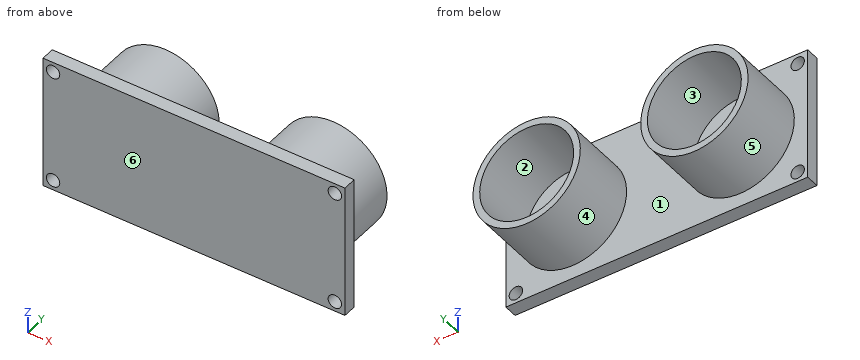
```python
from build123d import *

# Parameters (mm, degrees)
SKETCH1_W           = 45
SKETCH1_H           = 20
SKETCH1_R           = 1
SKETCH1_R_2         = 8
SKETCH1_R_3         = 7
BOSS_EXTRUDE1_DEPTH = 2
SKETCH2_R           = 8
SKETCH2_R_2         = 7
BOSS_EXTRUDE2_DEPTH = 12


with BuildPart() as part:
    # Sketch1 → Boss-Extrude1 (new body)
    with BuildSketch(Plane(origin=(0, 0, 0), x_dir=(1, 0, 0), z_dir=(0, 1, 0))):
        Rectangle(SKETCH1_W, SKETCH1_H)
        with Locations(Location((-21, -8.5, 0), (0, 0, 270))):
            Circle(SKETCH1_R, mode=Mode.SUBTRACT)
        with Locations(Location((-21, 8.5, 0), (0, 0, 270))):
            Circle(SKETCH1_R, mode=Mode.SUBTRACT)
        with Locations((-12.5, 0)):
            Circle(SKETCH1_R_2, mode=Mode.SUBTRACT)
        with Locations(Location((21, -8.5, 0), (0, 0, 270))):
            Circle(SKETCH1_R, mode=Mode.SUBTRACT)
        with Locations(Location((21, 8.5, 0), (0, 0, 270))):
            Circle(SKETCH1_R, mode=Mode.SUBTRACT)
        with Locations((12.5, 0)):
            Circle(SKETCH1_R_2, mode=Mode.SUBTRACT)
        with Locations((-12.5, 0)):
            Circle(SKETCH1_R_2)
        with Locations((-12.5, 0)):
            Circle(SKETCH1_R_3, mode=Mode.SUBTRACT)
        with Locations((-12.5, 0)):
            Circle(SKETCH1_R_3)
        with Locations((12.5, 0)):
            Circle(SKETCH1_R_2)
        with Locations((12.5, 0)):
            Circle(SKETCH1_R_3, mode=Mode.SUBTRACT)
        with Locations((12.5, 0)):
            Circle(SKETCH1_R_3)
    extrude(amount=BOSS_EXTRUDE1_DEPTH)

    # Sketch2 → Boss-Extrude2 (add)
    with BuildSketch(Plane(origin=(0, 0, 0), x_dir=(1, 0, 0), z_dir=(0, 1, 0))):
        with Locations(Location((-12.5, 0, 0), (0, 0, 270))):
            Circle(SKETCH2_R)
        with Locations(Location((-12.5, 0, 0), (0, 0, 270))):
            Circle(SKETCH2_R_2, mode=Mode.SUBTRACT)
        with Locations(Location((12.5, 0, 0), (0, 0, 270))):
            Circle(SKETCH2_R)
        with Locations(Location((12.5, 0, 0), (0, 0, 270))):
            Circle(SKETCH2_R_2, mode=Mode.SUBTRACT)
    extrude(amount=BOSS_EXTRUDE2_DEPTH)


solid = part.part
```
Read the model definition and answer for the solid it produces. Units are mm, in the model's axes. Face numbers are marked on the shaded views. A direction names the side the tool comes from. Coordinates: 2 decimals unless noted, no trailing zeros. Loops run counter-clockwise (first coordinate to the right, second up) from the corner with the lowest first, then second, coordinate; pieces in that order, holes last.
(1) The mould has two halves that part along Z. Classify the marked faces 1, 2, 3 and 4: released by +Z, released by -Z, zero draft, split by the parting line, or undercut.
Solution:
face 1: zero draft
face 2: undercut
face 3: undercut
face 4: split by the parting line
(2) The part is cut by section D-D (z = 0). Determine the outline of the cut face in (x, y).
Solution:
outline: (-22.5, 0) - (22.5, 0) - (22.5, 2) - (20.5, 2) - (20.5, 12) - (19.5, 12) - (19.5, 2) - (5.5, 2) - (5.5, 12) - (4.5, 12) - (4.5, 2) - (-4.5, 2) - (-4.5, 12) - (-5.5, 12) - (-5.5, 2) - (-19.5, 2) - (-19.5, 12) - (-20.5, 12) - (-20.5, 2) - (-22.5, 2) - close
(3) Flat-ended cylindrical pins translate along their axes: pin 1 Ø8.5 at (x, z) = (12.5, 0) entering from -Y; pin 2 Ø3 at (x, y) = (-10.5, 5.5) entering from -Z; pin 3 Ø2.5 at (x, z) = (21, 8.5) entering from +Y; pin 4 Ø4 at (y, z) = (8, 1.5) entering from -X. Find the tip coordinate at first contact, or state that the pin passes through.
Solution:
pin 1: stops at y = 0
pin 2: stops at z = -7.98
pin 3: stops at y = 2
pin 4: stops at x = -20.5
(4) A tool of negligible diameter and unlimited length cuts with its end or side. For the marked faces 5 and 6, from which of +Z, -Z, +X, -X, +Y, -Y can it reach the whole face along a straight path? Write none if from no direction.
Solution:
face 5: +Y
face 6: +Z, -Z, +X, -X, -Y
(5) The part is cut by section B-B (x = -21). Determine the outline of the cut face in (y, z), and give its area (3 significant figures).
Solution:
outline: (0, -10) - (2, -10) - (2, -9.5) - (0, -9.5) - close; (0, -7.5) - (2, -7.5) - (2, 7.5) - (0, 7.5) - close; (0, 9.5) - (2, 9.5) - (2, 10) - (0, 10) - close
area: 32.0 mm2
(6) Consider line 1 along X through (y, z) = (8.75, 0.25); line 2 along X through (y, z) = (0.5, -8.5); line 3 along Z through (x, y) = (12.5, 9.5). Determine where each line is inside the solid, lowest interval first.
Solution:
line 1: x = -20.5 to -19.5, -5.5 to -4.5, 4.5 to 5.5, 19.5 to 20.5
line 2: x = -22.5 to -22, -20 to 20, 22 to 22.5
line 3: z = -8 to -7, 7 to 8
(7) The part is cut by section A-A (z = 8.5). Determine the outline of the cut face in (x, y).
Solution:
outline: (-22.5, 0) - (-22, 0) - (-22, 2) - (-22.5, 2) - close; (-20, 0) - (20, 0) - (20, 2) - (-20, 2) - close; (22, 0) - (22.5, 0) - (22.5, 2) - (22, 2) - close
(8) The part is cut by section C-C (y = 11). Determine the outline of the cut face in (x, z), and give its area (3 significant figures).
Solution:
outline: circle Ø16 at (-12.5, 0); circle Ø16 at (12.5, 0); hole circle Ø14 at (-12.5, 0); hole circle Ø14 at (12.5, 0)
area: 94.2 mm2
